Build history of the part. All positions in model axes, mm. Face numbers are marked on the shaded views. A direction names the side the tool comes from. Round coordinates to 2 decimals unless told otherwise and drop trailing zeros. Loops run counter-clockwise (first coordinate to the right, second up) from the corner with the lowest first, then second, coordinate; pieces in that order, holes last. Notation, with made-up numbers: M 50,89.25 L 64,89.25 A31 cw 64,119.25 Z; hole C 43.5,41 d11. An arc over 180 degrees is marked long. One line per item, written item: value.
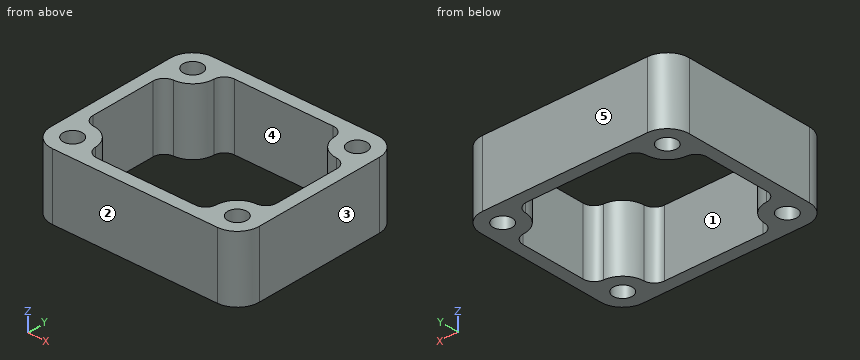
```python
from build123d import *

# Parameters (mm, degrees)
SKETCH_R  = 1.75
PAD_DEPTH = 12
FILLET_R  = 2


with BuildPart() as part:
    # Sketch → Pad (new body)
    with BuildSketch(Plane.XY):
        with BuildLine():
            Line((-15, 16), (15, 16))
            ThreePointArc((19, 12), (17.828427, 14.828427), (15, 16))
            Line((19, 12), (19, -12))
            ThreePointArc((15, -16), (17.828427, -14.828427), (19, -12))
            Line((15, -16), (-15, -16))
            ThreePointArc((-19, -12), (-17.828427, -14.828427), (-15, -16))
            Line((-19, -12), (-19, 12))
            ThreePointArc((-15, 16), (-17.828427, 14.828427), (-19, 12))
        make_face()
        with Locations((-15, 12)):
            Circle(SKETCH_R, mode=Mode.SUBTRACT)
        with Locations((15, 12)):
            Circle(SKETCH_R, mode=Mode.SUBTRACT)
        with Locations((15, -12)):
            Circle(SKETCH_R, mode=Mode.SUBTRACT)
        with Locations((-15, -12)):
            Circle(SKETCH_R, mode=Mode.SUBTRACT)
        with BuildLine():
            Line((-16.75, 8), (-15, 8))
            ThreePointArc((-15, 8), (-12.171573, 9.171573), (-11, 12))
            Line((-11, 12), (-11, 13.75))
            Line((-11, 13.75), (11, 13.75))
            Line((11, 13.75), (11, 12))
            ThreePointArc((11, 12), (12.171573, 9.171573), (15, 8))
            Line((15, 8), (16.75, 8))
            Line((16.75, 8), (16.75, -8))
            Line((15, -8), (16.75, -8))
            ThreePointArc((15, -8), (12.171573, -9.171573), (11, -12))
            Line((11, -13.75), (11, -12))
            Line((11, -13.75), (-11, -13.75))
            Line((-11, -12), (-11, -13.75))
            ThreePointArc((-11, -12), (-12.171573, -9.171573), (-15, -8))
            Line((-16.75, -8), (-15, -8))
            Line((-16.75, -8), (-16.75, 8))
        make_face(mode=Mode.SUBTRACT)
    extrude(amount=PAD_DEPTH)

    # Fillet
    fillet_edges = [part.edges().sort_by_distance(p)[0] for p in [
        (-11, 13.75, 6),
        (-16.75, 8, 6),
        (11, 13.75, 6),
        (16.75, 8, 6),
        (16.75, -8, 6),
        (11, -13.75, 6),
        (-11, -13.75, 6),
        (-16.75, -8, 6),
    ]]
    fillet(fillet_edges, radius=FILLET_R)


solid = part.part
```
Item 1: Drop a flat-ended pin along its axis: P1, Ø3, axis at x = -15, y = 12, coming from the +Z side. Give the stop position or say it passes through.
Check values:
P1: passes through
Item 2: Pull direction X, two halves, no side cores. Call the marked faces 1, 2 and 3: pulls with the +X half, pulls with the -X half, needs draft (parallel to the pull), parting line crosses it, or undercut.
Check values:
face 1: undercut
face 2: needs draft
face 3: pulls with the +X half
Item 3: Which spindle directions (+Z, -Z, +X, -X, +Y, -Y) get a long thin tool onto all of the face, cutting with end or side? Do the marked faces 4 and 5. Say none if no direction does.
Check values:
face 4: +Z, -Z
face 5: +Z, -Z, +X, -X, +Y
Item 4: Slice it at C-C, the plane z = 7.5. Give the number of separate pieces and of enclosed holes in the cut face, and give its area (3 significant figures).
Check values:
separate pieces: 1
enclosed holes: 5
area: 368 mm2
Item 5: Slice it at B-B, the plane x = -8.5. Give the cut face in (y, z), and give its area (3 significant figures).
Check values:
outline: M -16,0 L -13.75,0 L -13.75,12 L -16,12 Z; M 13.75,0 L 16,0 L 16,12 L 13.75,12 Z
area: 54.0 mm2
Item 6: Wall check: line 1 along Y through (x, z) = (0.5, 10); line 2 along X through (y, z) = (-3.5, 8.5); line 3 along X through (y, z) = (10.5, 4). Give the ranges that are in metal, low to high.
Check values:
line 1: y = -16 to -13.75, 13.75 to 16
line 2: x = -19 to -16.75, 16.75 to 19
line 3: x = -19 to -15.9, -14.1 to -11.29, 11.29 to 14.1, 15.9 to 19
Item 7: Slice it at A-A, the plane y = 0. Give the cut face in (x, z).
Check values:
outline: M -19,0 L -16.75,0 L -16.75,12 L -19,12 Z; M 16.75,0 L 19,0 L 19,12 L 16.75,12 Z
